Autodesk Inventor part; units mm, degrees
ref_plane "YZ Plane" through (0, 0, 0) normal (1, 0, 0) x (0, 1, 0)
ref_plane "XZ Plane" through (0, 0, 0) normal (0, 1, 0) x (-1, 0, 0)
ref_plane "XY Plane" through (0, 0, 0) normal (0, 0, 1) x (1, 0, 0)
sketch "스케치1" plane through (0, 0, 0) normal (1, 0, 0) x (0, 1, 0)
  line L0 (21.75, 7) -> (-21.75, 7)
  line L1 (-21.75, 7) -> (-21.75, 0)
  line L2 (-21.75, 0) -> (-3.25, 0)
  line L3 (-3.25, 0) -> (-3.25, 0)
  line L4 (-3.25, 0) -> (21.75, 0)
  line L5 (21.75, 0) -> (21.75, 7)
  point P0 (0, 0)
  point P1 (0, 7)
  dimension "d0" = 43.5
  dimension "d1" = 25
  dimension "d2" = 7
  dimension "d3" = 7
extrude "돌출1" add sketch "스케치1" along normal mid plane 27.14
sketch "스케치2" plane through (13.57, 21.75, 0) normal (0, 0, -1) x (-1, 0, 0)
  circle A0 centre (8.57, -9) radius 1.05
  circle A1 centre (18.57, -9) radius 1.05
  circle A2 centre (8.57, -34.5) radius 1.05
  circle A3 centre (18.57, -34.5) radius 1.05
  line L0 (8.57, -9) -> (18.57, -9) construction
  line L1 (8.57, -34.5) -> (18.57, -34.5) construction
  line L2 (27.14, -43.5) -> (0, -43.5)
  point P0 (13.57, -21.75)
  point P1 (13.57, -34.5)
  point P2 (13.57, -9)
  dimension "d41" = 2.1
  dimension "d42" = 2.1
  dimension "d43" = 2.1
  dimension "d44" = 2.1
  dimension "d45" = 25.5
  dimension "d46" = 9
  dimension "d47" = 10
  dimension "d48" = 10
extrude "돌출2" cut sketch "스케치2" against normal through all
sketch "스케치3" plane through (13.57, 21.75, 0) normal (0, 0, -1) x (-1, 0, 0)
  circle A0 centre (18.57, -34.5) radius 1.05
  circle A1 centre (18.57, -9) radius 1.05
  circle A2 centre (8.57, -34.5) radius 1.05
  circle A3 centre (8.57, -9) radius 1.05
  line L0 (27.14, 0) -> (0, 0)
  line L1 (0, -43.5) -> (0, 0)
  line L2 (27.14, -43.5) -> (0, -43.5)
  line L3 (27.14, 0) -> (27.14, -43.5)
  circle A4 centre (8.57, -9) radius 1.05
  circle A5 centre (8.57, -9) radius 2.25
  circle A6 centre (18.57, -9) radius 2.25
  circle A7 centre (8.57, -34.5) radius 1.05
  circle A8 centre (8.57, -34.5) radius 2.25
  circle A9 centre (18.57, -34.5) radius 2.25
  point P0 (13.57, -21.75)
  dimension "d51" = 4.5
  dimension "d52" = 4.5
  dimension "d53" = 4.5
  dimension "d54" = 4.5
extrude "돌출3" cut sketch "스케치3" against normal blind 4 contours A5 | A6 | A8 | A9
sketch "스케치4" plane through (-13.57, -21.75, 0) normal (0, -1, 0) x (1, 0, 0)
  circle A0 centre (13.57, -2.7) radius 5.25
  line L0 (0, 0) -> (27.14, 0)
  line L1 (0, 0) -> (27.14, 0)
  point P0 (13.57, 0)
  point P1 (13.57, 0)
  point P2 (13.57, 0)
  dimension "d67" = 10.5
  dimension "d68" = 2.7
extrude "돌출4" cut sketch "스케치4" against normal through all
sketch "스케치5" plane through (13.57, -21.75, 0) normal (0, 0, -1) x (-1, 0, 0)
  line L0 (9.0675, 0) -> (9.0675, 6.8057)
  arc A0 (9.0675, 11.1943) -> (9.0675, 6.8057) centre (8.57, 9) ccw
  line L1 (9.0675, 11.1943) -> (9.0675, 32.3057)
  arc A1 (9.0675, 36.6943) -> (9.0675, 32.3057) centre (8.57, 34.5) ccw
  line L2 (9.0675, 36.6943) -> (9.0675, 43.5)
  line L3 (9.0675, 43.5) -> (0, 43.5)
  line L4 (0, 0) -> (0, 43.5)
  line L5 (9.0675, 0) -> (0, 0)
  circle A2 centre (3.4, 26.75) radius 1.4
  circle A3 centre (3.4, 16.75) radius 1.4
  line L6 (9.0675, 0) -> (0, 0)
  point P0 (13.57, 21.75)
  point P1 (4.5338, 0)
  point P2 (4.5338, 0)
  dimension "d71" = 2.8
  dimension "d72" = 2.8
  dimension "d78" = 3.4
  dimension "d79" = 26.75
  dimension "d80" = 16.75
extrude "돌출5" cut sketch "스케치5" against normal blind 5 contours A2 | A3
mirror "미러1" about plane through (0, 0, 0) normal (1, 0, 0) of "돌출5"
fillet "모깎기2" radius 2 2 edges at (13.57, 21.75, 3.5) (-13.57, 21.75, 3.5)
ref_plane "작업 평면1" through (0, 0, 0) normal (1, 0, 0) x (0, 1, 0)
properties part number "end_arm_수정"
Here's how the part is built. I have some questions about the finished solid (model axes, mm). A direction names the side the tool comes from. Coordinates: 2 decimals unless noted, no trailing zeros. Order: outer loops, then holes, each group sorted by start corner. A loop starts at its lowest first (then second) coordinate and runs counter-clockwise, first axis right, second up. Notation, with made-up numbers: M 8,53 L 65,53 A32 cw 65,85 Z; hole C 84.5,40 d5. An arc over 180 degrees is marked long. Answer as a JSON object with one key per item and string values. Group by question number.
(1) If we mould it in two halves opening along X, with no side actions, what happens to faces 3 (the face through (0, 0, 7)), 4 (the face through (-13.57, -1, 4)), 5 (the face through (5, -14, 4)), 6 (the face through (10.473, -6.367, 2.465))? For each: released by +X, released by -X, zero draft, split by the parting line, or undercut.
(2) Suppose I cut it at B-B, the plane y = -12.75. Please give me the cut outline in (x, z), then the cut area to 3 significant figures.
(3) Suppose I cut it at A-A, the plane x = -5. Please give me the cut outline in (y, z), then the cut area to 3 significant figures.
(4) Suppose I cut it at C-C, the plane x = -10.17. Please give me the cut outline in (y, z).
(5) Which directions (+Z, -Z, +X, -X, +Y, -Y) give clear straight access to the entire face, cutting with the end or side of a thin tool? Please do faces 1 (the face through (13.57, -1, 4)), 2 (the face through (-10, 5, 5)).
(6) Suppose I cut it at D-D, the plane y = -5. Please give me the cut outline in (x, z), then the cut area to 3 significant figures.
(7) For pin 1 (6 mm diameter, centred on x = -5, y = 2.5, fed in from -Z); pin 2 (2.5 mm diameter, centred on x = -5, y = 12.75, fed in from -Z); pin 3 (0.8 mm diameter, centred on x = 10.5, y = -5, fed in from -Z), each with a flat end and sliding along its axis, tell me the tip position at first contact or that it passes through.
(8) I need wall thicknesses on probe 1 along Y at (x, z) = (5, 5.95); probe 2 along Y at (x, z) = (10.17, 2); probe 3 along X at (y, z) = (12.75, 1.4). Which ranges of each line are inside material? Lowest first, please.
Values found:
{
 "1": {"face 3": "zero draft", "face 4": "released by -X", "face 5": "undercut", "face 6": "undercut"},
 "2": {"outline": "M -13.57,0 L -7.25,0 L -7.25,4 L -6.05,4 L -6.05,7 L -13.57,7 Z; M -3.95,4 L -2.75,4 L -2.75,1.77 A5.25 cw 2.75,1.77 L 2.75,4 L 3.95,4 L 3.95,7 L -3.95,7 Z; M 6.05,4 L 7.25,4 L 7.25,0 L 13.57,0 L 13.57,7 L 6.05,7 Z", "area": "129 mm^2"},
 "3": {"outline": "M -21.75,0 L -15,0 L -15,4 L -13.8,4 L -13.8,7 L -21.75,7 Z; M -11.7,4 L -10.5,4 L -10.5,0 L 10.5,0 L 10.5,4 L 11.7,4 L 11.7,7 L -11.7,7 Z; M 13.8,4 L 15,4 L 15,0 L 21.75,0 L 21.75,7 L 13.8,7 Z", "area": "256 mm^2"},
 "4": {"outline": "M -21.75,0 L -6.4,0 L -6.4,5 L -3.6,5 L -3.6,0 L 3.6,0 L 3.6,5 L 6.4,5 L 6.4,0 L 21.75,0 L 21.75,7 L -21.75,7 Z"},
 "5": {"face 1": "+Z, -Z, +X, +Y, -Y", "face 2": "-Z"},
 "6": {"outline": "M -13.57,0 L -11.57,0 L -11.57,5 L -8.77,5 L -8.77,0 L -4.5,0 A5.25 cw 4.5,0 L 8.77,0 L 8.77,5 L 11.57,5 L 11.57,0 L 13.57,0 L 13.57,7 L -13.57,7 Z", "area": "146 mm^2"},
 "7": {"pin 1": "stops at z = 0", "pin 2": "stops at z = 4", "pin 3": "stops at z = 5"},
 "8": {"probe 1": "y = -21.75 to -13.8, -11.7 to 11.7, 13.8 to 21.75", "probe 2": "y = -21.75 to -6.4, -3.6 to 3.6, 6.4 to 21.75", "probe 3": "x = -13.57 to -7.25, 7.25 to 13.57"}
}
